The listing builds one solid part. Answer for the finished solid, in the listing's coordinates (mm). A direction names the side the tool comes from. Give positions to 0.01 mm unless a question says otherwise; leave off trailing zeros. Loops run counter-clockwise (first coordinate to the right, second up) from the corner with the lowest first, then second, coordinate; pieces in that order, holes last. Notation, with made-up numbers: (-15.5, 82) - (34.5, 82) arc R35 cw to (34.5, 114) - close; hole circle Ø6 at (7, -12.75). An arc over 180 degrees is marked (long way). Write item = value, one per line. Start each with the question number.
1) Flat-ended cylindrical pins translate along their axes: P1, Ø5, axis at y = 7, z = 6, coming from the +X side; P2, Ø3.5, axis at x = 18.5, z = 12.5, coming from the +Y side; P3, Ø4, axis at x = 6, y = 0, coming from the +Z side; P4, Ø8, axis at x = -14.5, z = 6, coming from the +Y side. Find the tip coordinate at first contact, or state that the pin passes through.
2) The part is cut by section A-A on x = -18.55. Write down the section's boundary in (y, z) (3 decimals).
3) Consider probe 1 along Z at (x, y) = (-18.55, -12.1) (3 decimals); probe 2 along X at (y, z) = (-8, 20.5); probe 3 along Y at (x, z) = (-15.5, 21.5). Determine where each line is inside the solid, lowest interval first.
4) The part is cut by section D-D on y = 7. Write down the section's boundary in (x, z).
5) The mould has two halves that part along Z. Classify faces 4 (the flat face through (-11, 6, 17)), 5 (the flat face through (-10, -1, 0)), 6 (the flat face through (9.1, -1, 12)): +Z half, -Z half, draft (parallel to the pull), parting line (faces both ways), or undercut.
6) The part is cut by section C-C on z = 8.5. Write down the section's boundary in (x, y).
7) The part is cut by section B-B on y = -1.5. Write down the section's boundary in (x, z).
8) Which of the six approach directions +Z, -Z, +X, -X, +Y, -Y give full straight-line access (tool end or side, diameter ignored) to faces 1 (the flat face through (-19, -11, 7)), 2 (the flat face through (-9.1, -13, 7)), 3 (the flat face through (-11, -6, 15.2))?
from build123d import *

# Parameters (mm, degrees)
BOSS_EXTRUDE1_DEPTH     = 23.85
CUT_EXTRUDE2_DEPTH      = 12
CUT_EXTRUDE2_DEPTH_BACK = 10
SKETCH2_W               = 3.2
SKETCH2_H               = 20
SKETCH4_R               = 1.45
CUT_EXTRUDE3_DEPTH      = 10


with BuildPart() as part:
    # Sketch1 → Boss-Extrude1 (new body)
    with BuildSketch(Plane.XY):
        with BuildLine():
            Line((-9.1, -10.52892562), (-9.1, 11))
            Line((-9.1, 11), (9.1, 11))
            Line((9.1, 11), (9.1, -11))
            Line((9.1, -11), (9.1, -14))
            Line((9.1, -14), (12.1, -14))
            Line((12.1, -14), (22, -14))
            Line((22, -14), (22, -11))
            Line((22, -11), (15.1, -11))
            ThreePointArc((15.1, -11), (12.978679656, -10.121320344), (12.1, -8))
            Line((12.1, -8), (12.1, 11))
            ThreePointArc((12.1, 11), (11.221320344, 13.121320344), (9.1, 14))
            Line((9.1, 14), (-9.1, 14))
            ThreePointArc((-9.1, 14), (-11.221320344, 13.121320344), (-12.1, 11))
            Line((-12.1, 11), (-12.1, -8))
            ThreePointArc((-12.1, -8), (-12.978679656, -10.121320344), (-15.1, -11))
            Line((-15.1, -11), (-22, -11))
            Line((-22, -11), (-22, -14))
            Line((-22, -14), (-12.1, -14))
            Line((-12.1, -14), (-9.1, -14))
            Line((-9.1, -14), (-9.1, -11))
            Line((-9.1, -11), (-9.507142857, -11))
            Line((-9.507142857, -11), (-9.1, -10.52892562))
        make_face()
    extrude(amount=BOSS_EXTRUDE1_DEPTH)

    # Sketch2 → Cut-Extrude2 (cut, two sides: drawn at the far end of the back side and taken through both)
    with BuildSketch(Plane.ZY.offset(12.1).offset(-CUT_EXTRUDE2_DEPTH_BACK)):
        with Locations((16.8, -4)):
            Rectangle(SKETCH2_W, SKETCH2_H)
    extrude(amount=CUT_EXTRUDE2_DEPTH + CUT_EXTRUDE2_DEPTH_BACK, mode=Mode.SUBTRACT)

    # Sketch4 → Cut-Extrude3 (cut)
    with BuildSketch(Plane(origin=(0, -11, 0), x_dir=(1, 0, 0), z_dir=(0, 1, 0))):
        with Locations(Location((-18.55, -21.125, 0), (0, 0, 180))):
            Circle(SKETCH4_R)
        with Locations(Location((-18.55, -2.725, 0), (0, 0, 180))):
            Circle(SKETCH4_R)
        with Locations(Location((18.55, -21.125, 0), (0, 0, 270))):
            Circle(SKETCH4_R)
        with Locations(Location((18.55, -2.725, 0), (0, 0, 180))):
            Circle(SKETCH4_R)
    extrude(amount=-CUT_EXTRUDE3_DEPTH, mode=Mode.SUBTRACT)


solid = part.part
Answer below:
q1.P1 = 12.1
q1.P2 = -11
q1.P3 = through
q1.P4 = 13.65
q2.outline = (-14, 0) - (-11, 0) - (-11, 1.275) - (-14, 1.275) - close; (-14, 4.175) - (-11, 4.175) - (-11, 15.2) - (-14, 15.2) - close; (-14, 18.4) - (-11, 18.4) - (-11, 19.675) - (-14, 19.675) - close; (-14, 22.575) - (-11, 22.575) - (-11, 23.85) - (-14, 23.85) - close
q3.probe_1 = 0 to 1.275, 4.175 to 15.2, 18.4 to 19.675, 22.575 to 23.85
q3.probe_2 = -12.1 to -9.1, 9.1 to 12.1
q3.probe_3 = -14 to -11
q4.outline = (-12.1, 0) - (-9.1, 0) - (-9.1, 23.85) - (-12.1, 23.85) - close; (9.1, 0) - (12.1, 0) - (12.1, 23.85) - (9.1, 23.85) - close
q5.face_4 = undercut
q5.face_5 = -Z half
q5.face_6 = draft
q6.outline = (-22, -14) - (-9.1, -14) - (-9.1, -11) - (-9.51, -11) - (-9.1, -10.53) - (-9.1, 11) - (9.1, 11) - (9.1, -14) - (22, -14) - (22, -11) - (15.1, -11) arc R3 cw to (12.1, -8) - (12.1, 11) arc R3 ccw to (9.1, 14) - (-9.1, 14) arc R3 ccw to (-12.1, 11) - (-12.1, -8) arc R3 cw to (-15.1, -11) - (-22, -11) - close
q7.outline = (-12.1, 0) - (-9.1, 0) - (-9.1, 15.2) - (-12.1, 15.2) - close; (-12.1, 18.4) - (-9.1, 18.4) - (-9.1, 23.85) - (-12.1, 23.85) - close; (9.1, 0) - (12.1, 0) - (12.1, 23.85) - (9.1, 23.85) - close
q8.face_1 = +Z, -Z, -X, +Y
q8.face_2 = +Z, -Z, -Y
q8.face_3 = -X, -Y
